Geometry: final body of the model. Coordinates: model frame, mm. A direction names the side the tool comes from. Give positions to 0.01 mm unless a question says otherwise; leave off trailing zeros. Write each loop counter-clockwise with the first axis right and the second up, starting at its lowest first coordinate (ties: lowest second). Pieces come first, ordered by that corner, then holes. Notation, with made-up numbers: M 35.5,42.5 L 67.5,42.5 A28 cw 67.5,77.5 Z; hole C -5,15.25 d7. An arc over 180 degrees is marked long. Use a Markdown table: item, result. Add a question column.
1) Section A-A on z = 8. Return the cut outline in (x, y), then the cut area to 3 significant figures.
2) Section B-B on x = 1.5. Return the cut outline in (y, z).
3) Pin query (flat end, axial travel): pin 1 (1 mm diameter, centred on x = 2, z = 6, fed in from -Y); pin 2 (0.7 mm diameter, centred on y = -4.5, z = 34, fed in from -X); pin 3 (5.5 mm diameter, centred on x = -2.5, y = 1, fed in from +Z). Return the tip coordinate at first contact, or that it passes through.
4) Draft query along Y for faces 1 (the flat face through (-0.49, -3.18, 28.64)), 2 (the flat face through (-1, 4, 14)), 3 (the flat face through (-0.5, -2.4, 19.7)). Return one class per face: +Y half, -Y half, draft (parallel to the pull), parting line (faces both ways), or undercut.
5) Line query: line 1 (Y direction, x = 0, z = 4); line 2 (Z direction, x = -0.75, y = 1.75). Output: solid intervals per line, ascending.
6) Set-up query: faces 4 (the flat face through (-1, 6.6, 35.9)), 5 (the flat face through (3, 7, 37)), 6 (the cylindrical face through (-3, 0, 5)), 7 (the flat face through (-0.493, -3.537, 22.558)). Return all of +Z, -Z, +X, -X, +Y, -Y with unobstructed straight access to the full face (end or side cutting, diameter ignored); none if empty.
```python
from build123d import *

# Parameters (mm, degrees)
F0_W         = 14
F0_H         = 14
F0_R         = 3
F1_DEPTH     = 10
F3_DEPTH     = 7
F5_DEPTH     = 1
F6_T1_DEPTH  = 7
F6_T6_DEPTH  = 7
F6_S7_R      = 6.75
F6_T8_DEPTH  = 6
F6_T12_DEPTH = 7
F6_S13_R     = 6.75
F6_T14_DEPTH = 6
F6_T18_DEPTH = 16.4948974278
F6_S20_R     = 6.75
F6_T21_DEPTH = 10
F7_R         = 5
F8_SIZE      = 2


# Not quite as in the source:
# - a fillet or chamfer that OpenCascade refuses, or shapes differently, is made with other operations: its cross-section is extruded or revolved along the edge and cut away or added


with BuildPart() as f1:
    # F0 (on Top) → F1 (new body)
    with BuildSketch(Plane.XY):
        Rectangle(F0_W, F0_H)
        Circle(F0_R, mode=Mode.SUBTRACT)
    extrude(amount=F1_DEPTH)

    # F2 (on face) → F3 (join)
    with BuildSketch(Plane.YZ.offset(7)):
        with BuildLine():
            Line((7, 31), (7, 40))
            ThreePointArc((7, 40), (-5.3648184804, 33.4918351342), (-7, 19.6148351929))
            ThreePointArc((-7, 19.6148351929), (-1.4918351342, 12.6351815196), (7, 10))
            Line((7, 10), (7, 19))
            Line((7, 19), (7, 22.75))
            ThreePointArc((7, 22.75), (4.75, 25), (7, 27.25))
            Line((7, 27.25), (7, 31))
        make_face()
        with BuildLine():
            ThreePointArc((7, 19), (13, 25), (7, 31))
            Line((7, 31), (7, 27.25))
            ThreePointArc((7, 27.25), (8.5909902577, 26.5909902577), (9.25, 25))
            ThreePointArc((9.25, 25), (8.5909902577, 23.4090097423), (7, 22.75))
            Line((7, 22.75), (7, 19))
        make_face()
        with BuildLine():
            ThreePointArc((7, 10), (-1.4918351342, 12.6351815196), (-7, 19.6148351929))
            Line((-7, 19.6148351929), (-7, 10))
            Line((-7, 10), (7, 10))
        make_face()
    extrude(amount=-F3_DEPTH)

    # F4 (on face) → F5 (join)
    with BuildSketch(Plane(origin=(0, 0, 0), x_dir=(0, -1, 0), z_dir=(-1, 0, 0))):
        with BuildLine():
            Line((-5.6015252753, 39.9346666667), (-7, 40))
            Line((-7, 40), (-7, 31.75))
            ThreePointArc((-7, 31.75), (-6.7748747563, 31.7462447795), (-6.55, 31.7349832962))
            Line((-6.55, 31.7349832962), (-5.6015252753, 39.9346666667))
        make_face()
        with BuildLine():
            Line((-1.4505915023, 38.9357118701), (-2.7740116474, 39.3923946042))
            Line((-2.7740116474, 39.3923946042), (-5.0983052413, 31.4765775719))
            ThreePointArc((-5.0983052413, 31.4765775719), (-4.8833571197, 31.4095493537), (-4.6707640976, 31.3353894995))
            Line((-4.6707640976, 31.3353894995), (-1.4505915023, 38.9357118701))
        make_face()
        with BuildLine():
            Line((2.2507621978, 36.8077685766), (1.1096122618, 37.6188029925))
            Line((1.1096122618, 37.6188029925), (-3.3506744822, 30.6784613466))
            ThreePointArc((-3.3506744822, 30.6784613466), (-3.1633173011, 30.5535903583), (-2.9802290354, 30.4225401236))
            Line((-2.9802290354, 30.4225401236), (2.2507621978, 36.8077685766))
        make_face()
        with BuildLine():
            Line((5.2026741611, 33.7232300966), (4.3362436153, 34.8229110092))
            Line((4.3362436153, 34.8229110092), (-1.8986903731, 29.4203099541))
            ThreePointArc((-1.8986903731, 29.4203099541), (-1.7541026971, 29.2477125006), (-1.6153519103, 29.070388796))
            Line((-1.6153519103, 29.070388796), (5.2026741611, 33.7232300966))
        make_face()
        with BuildLine():
            Line((7.1659980359, 29.9319873933), (6.6444799303, 31.231225195))
            Line((6.6444799303, 31.231225195), (-0.8599840314, 27.8040513378))
            ThreePointArc((-0.8599840314, 27.8040513378), (-0.7698794941, 27.5977102382), (-0.6867069498, 27.3884787756))
            Line((-0.6867069498, 27.3884787756), (7.1659980359, 29.9319873933))
        make_face()
        with BuildLine():
            Line((7.9816769983, 25.7411844029), (7.8473216282, 27.1347225741))
            Line((7.8473216282, 27.1347225741), (-0.3187052673, 25.9606251583))
            ThreePointArc((-0.3187052673, 25.9606251583), (-0.2903836024, 25.7372569414), (-0.2695274455, 25.5130684097))
            Line((-0.2695274455, 25.5130684097), (7.9816769983, 25.7411844029))
        make_face()
        with BuildLine():
            Line((-0.3976107999, 23.5960922926), (7.5836295897, 21.4903350603))
            Line((7.5836295897, 21.4903350603), (7.8473216282, 22.8652774259))
            Line((7.8473216282, 22.8652774259), (-0.3187052673, 24.0393748417))
            ThreePointArc((-0.3187052673, 24.0393748417), (-0.3544609277, 23.8170754719), (-0.3976107999, 23.5960922926))
        make_face()
        with BuildLine():
            ThreePointArc((-0.8599840314, 22.1959486622), (-0.9569203061, 21.9927275126), (-1.0605804615, 21.7928524285))
            Line((-1.0605804615, 21.7928524285), (6.004103244, 17.5238178982))
            Line((6.004103244, 17.5238178982), (6.6444799303, 18.768774805))
            Line((6.6444799303, 18.768774805), (-0.8599840314, 22.1959486622))
        make_face()
        with BuildLine():
            ThreePointArc((-1.8986903731, 20.5796900459), (-2.0489540617, 20.4120108852), (-2.2047265709, 20.2494365871))
            Line((-2.2047265709, 20.2494365871), (3.3710617919, 14.1629765475))
            Line((3.3710617919, 14.1629765475), (4.3362436153, 15.1770889908))
            Line((4.3362436153, 15.1770889908), (-1.8986903731, 20.5796900459))
        make_face()
        with BuildLine():
            ThreePointArc((-3.3506744822, 19.3215386534), (-3.5420921143, 19.2029858501), (-3.737357215, 19.0908831407))
            Line((-3.737357215, 19.0908831407), (-0.1021814076, 11.6800863867))
            Line((-0.1021814076, 11.6800863867), (1.1096122618, 12.3811970075))
            Line((1.1096122618, 12.3811970075), (-3.3506744822, 19.3215386534))
        make_face()
        with BuildLine():
            ThreePointArc((-5.0983052413, 18.5234224281), (-5.3153692987, 18.4636004253), (-5.5343077738, 18.4110511993))
            Line((-5.5343077738, 18.4110511993), (-4.1342448465, 10.2762964102))
            Line((-4.1342448465, 10.2762964102), (-2.7740116474, 10.6076053958))
            Line((-2.7740116474, 10.6076053958), (-5.0983052413, 18.5234224281))
        make_face()
    extrude(amount=F5_DEPTH)

    # F6: fillet of radius 5 on 2 edges, made by hand

    # F6_s2 → F6_t1 (join)
    with BuildSketch(Plane.YZ):
        with BuildLine():
            ThreePointArc((7, 15.2020410289), (7.7359856729, 17.8132058682), (9.7272727273, 19.655658743))
            ThreePointArc((9.7272727273, 19.655658743), (8.4024892973, 19.1662170274), (7, 19))
            Line((7, 19), (7, 15.2020410289))
        make_face()
    extrude(amount=F6_T1_DEPTH)


with BuildPart() as f6_tool4:
    # F6_s5 → F6_t6 (new body)
    with BuildSketch(Plane.YZ.offset(7)):
        with BuildLine():
            ThreePointArc((7, 34.7979589711), (7.7359856729, 32.1867941318), (9.7272727273, 30.344341257))
            ThreePointArc((9.7272727273, 30.344341257), (8.4024892973, 30.8337829726), (7, 31))
            Line((7, 31), (7, 34.7979589711))
        make_face()
    extrude(amount=-F6_T6_DEPTH)

    # F6_s7 → F6_t8 (cut, symmetric)
    with BuildSketch(Plane.YZ.offset(3.5)):
        with Locations((7, 25)):
            Circle(F6_S7_R)
    extrude(amount=F6_T8_DEPTH, both=True, mode=Mode.SUBTRACT)


with BuildPart() as f1_1:
    add(f1.part)

    # F6_t3: union F6_tool4
    add(f6_tool4.part)


with BuildPart() as f6_tool10:
    # F6_s11 → F6_t12 (new body)
    with BuildSketch(Plane.YZ.offset(7)):
        with BuildLine():
            ThreePointArc((7, 34.7979589711), (7.7359856729, 32.1867941318), (9.7272727273, 30.344341257))
            ThreePointArc((9.7272727273, 30.344341257), (8.4024892973, 30.8337829726), (7, 31))
            Line((7, 31), (7, 34.7979589711))
        make_face()
    extrude(amount=-F6_T12_DEPTH)

    # F6_s13 → F6_t14 (intersect, symmetric)
    with BuildSketch(Plane.YZ.offset(3.5)):
        with Locations((7, 25)):
            Circle(F6_S13_R)
    extrude(amount=F6_T14_DEPTH, both=True, mode=Mode.INTERSECT)


with BuildPart() as f1_2:
    add(f1_1.part)

    # F6_t9: union F6_tool10
    add(f6_tool10.part)


with BuildPart() as f6_tool16:
    # F6_s17 → F6_t18 (new body)
    with BuildSketch(Plane.YZ.offset(7)):
        with BuildLine():
            ThreePointArc((7, 34.7979589711), (7.7359856729, 32.1867941318), (9.7272727273, 30.344341257))
            ThreePointArc((9.7272727273, 30.344341257), (8.4024892973, 30.8337829726), (7, 31))
            Line((7, 31), (7, 34.7979589711))
        make_face()
    extrude(amount=-F6_T18_DEPTH)

    split(bisect_by=Plane.YZ, keep=Keep.BOTTOM)

    # F6_s20 → F6_t21 (cut, symmetric)
    with BuildSketch(Plane.YZ.offset(-1.2)):
        with Locations((7, 25)):
            Circle(F6_S20_R)
    extrude(amount=F6_T21_DEPTH, both=True, mode=Mode.SUBTRACT)

    split(bisect_by=Plane.YZ.offset(-1), keep=Keep.TOP)


with BuildPart() as f1_3:
    add(f1_2.part)

    # F6_t15: union F6_tool16
    add(f6_tool16.part)

    # F7
    f7_edges = [f1_3.edges().sort_by_distance(p)[0] for p in [
        (-7, 7, 5),
        (-7, -7, 5),
    ]]
    fillet(f7_edges, radius=F7_R)

    # F8
    f8_edges = [f1_3.edges().sort_by_distance(p)[0] for p in [
        (7, 7, 22.75),
    ]]
    chamfer(f8_edges, length=F8_SIZE)


solid = f1_3.part
```
Found:
| question | item | result |
|---|---|---|
| 1 | outline | M -7,-2 A5 ccw -2,-7 L 7,-7 L 7,7 L -2,7 A5 ccw -7,2 Z; hole C 0,0 d6 |
| 1 | area | 157 mm² |
| 2 | outline | M -7,0 L -2.6,0 L -2.6,10 L 2.6,10 L 2.6,0 L 7,0 L 7,15.2 A5 cw 9.73,19.66 A6 ccw 9.73,30.34 A5 cw 7,34.8 L 7,40 A15 ccw -7,19.61 Z; hole C 7,25 d4.5 |
| 3 | pin 1 | y = -7 |
| 3 | pin 2 | x = -1 |
| 3 | pin 3 | z = 39.39 |
| 4 | face 1 | -Y half |
| 4 | face 2 | draft |
| 4 | face 3 | undercut |
| 5 | line 1 | -7 to -3, 3 to 7 |
| 5 | line 2 | 15.04 to 16.83, 19.75 to 20.45, 29.24 to 29.55, 31.92 to 33.17, 38.23 to 39.04 |
| 6 | face 4 | +Z, -X, +Y, -Y |
| 6 | face 5 | +Z, +X, -X, +Y |
| 6 | face 6 | -Z |
| 6 | face 7 | -X |
